Verification items for the finished model (mm, model axes). Face numbers are marked on the shaded views. A direction names the side the tool comes from. Give positions to 0.01 mm unless a question says otherwise; leave off trailing zeros. Write each loop counter-clockwise with the first axis right and the second up, starting at its lowest first coordinate (ties: lowest second). Pieces come first, ordered by that corner, then holes. Notation, with made-up numbers: M 38,-14.75 L 75,-14.75 A22 cw 75,5.25 Z; hole C 16,38.25 d6. An arc over 180 degrees is marked long. Answer as a JSON object with one key per item and string values.
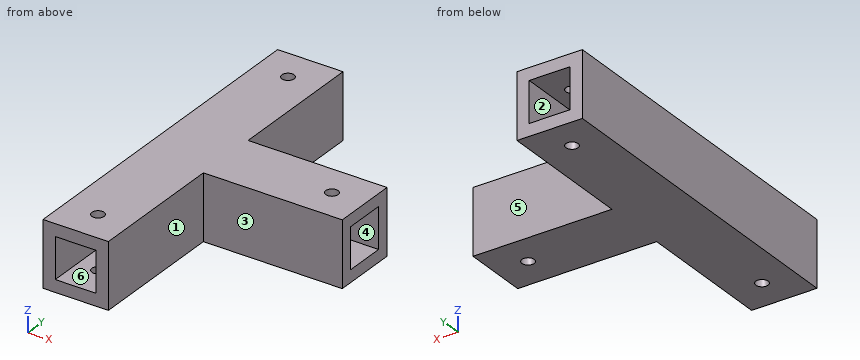
```python
from build123d import *

# Parameters (mm, degrees)
F0_W     = 16
F0_H     = 34
F1_DEPTH = 16
F2_W     = 10
F2_H     = 10
F3_DEPTH = 30
F4_W     = 10
F4_H     = 10
F5_DEPTH = 84
F6_R     = 1.5
F7_DEPTH = 16


with BuildPart() as f1:
    # F0 (on Top) → F1 (new body)
    with BuildSketch(Plane.XY):
        with Locations((-17, 33)):
            Rectangle(F0_W, F0_H)
        Polygon((-9, 16), (-25, 16), (-25, 0), (-9, 0), (25, 0), (25, 16), align=None)
        with Locations((-17, -17)):
            Rectangle(F0_W, F0_H)
    extrude(amount=F1_DEPTH)

    # F2 (on face) → F3 (cut)
    with BuildSketch(Plane.YZ.offset(25)):
        with Locations((8, 8)):
            Rectangle(F2_W, F2_H)
    extrude(amount=-F3_DEPTH, mode=Mode.SUBTRACT)

    # F4 (on face) → F5 (cut)
    with BuildSketch(Plane.XZ.offset(34)):
        with Locations((-17, 8)):
            Rectangle(F4_W, F4_H)
    extrude(amount=-F5_DEPTH, mode=Mode.SUBTRACT)

    # F6 (on face) → F7 (cut)
    with BuildSketch(Plane(origin=(0, 0, 0), x_dir=(1, 0, 0), z_dir=(0, 0, -1))):
        with Locations((-17, -42)):
            Circle(F6_R)
        with Locations((17, -8)):
            Circle(F6_R)
        with Locations((-17, 26)):
            Circle(F6_R)
    extrude(amount=-F7_DEPTH, mode=Mode.SUBTRACT)


solid = f1.part
```
1) Release check for a two-part mould opening along X. For the marked faces 1, 2 and 3 record: pulls with the +X half, pulls with the -X half, needs draft (parallel to the pull), parting line crosses it, or undercut.
Completed:
{"face 1": "pulls with the +X half", "face 2": "undercut", "face 3": "needs draft"}
2) Access from +Z, -Z, +X, -X, +Y, -Y to the whole of each face (thin tool, end or side, straight path). Record for the marked faces 4, 5 and 6.
Completed:
{"face 4": "+X", "face 5": "+Z, -Z, +X, +Y", "face 6": "+Y, -Y"}
3) Section check D-D on y = -3. Record the boundary of the cut face in (x, z), and give its area (3 significant figures).
Completed:
{"outline": "M -25,0 L -9,0 L -9,16 L -25,16 Z; hole M -22,3 L -12,3 L -12,13 L -22,13 Z", "area": "156 mm2"}
4) Section check B-B on y = 42. Record the boundary of the cut face in (x, z).
Completed:
{"outline": "M -25,0 L -18.5,0 L -18.5,3 L -22,3 L -22,13 L -18.5,13 L -18.5,16 L -25,16 Z; M -15.5,0 L -9,0 L -9,16 L -15.5,16 L -15.5,13 L -12,13 L -12,3 L -15.5,3 Z"}
5) Section check C-C on x = -17. Record the boundary of the cut face in (y, z), and give its area (3 significant figures).
Completed:
{"outline": "M -34,0 L -27.5,0 L -27.5,3 L -34,3 Z; M -34,13 L -27.5,13 L -27.5,16 L -34,16 Z; M -24.5,0 L 40.5,0 L 40.5,3 L -24.5,3 Z; M -24.5,13 L 40.5,13 L 40.5,16 L -24.5,16 Z; M 43.5,0 L 50,0 L 50,3 L 43.5,3 Z; M 43.5,13 L 50,13 L 50,16 L 43.5,16 Z", "area": "468 mm2"}
6) Go/stop test with flat-tipped pins: pin 1 (2.5 mm diameter, centred on x = -17, y = 42, fed in from -Z); pin 2 (4 mm diameter, centred on y = 40, z = 9.5, fed in from +X); pin 3 (5 mm diameter, centred on x = 12, z = 7, fed in from +Y); pin 4 (5 mm diameter, centred on y = 7, z = 7, fed in from +X). Record where each tip stops, or that it passes through.
Completed:
{"pin 1": "passes through", "pin 2": "stops at x = -9", "pin 3": "stops at y = 16", "pin 4": "stops at x = -5"}
7) Section check A-A on x = 17. Record the boundary of the cut face in (y, z).
Completed:
{"outline": "M 0,0 L 6.5,0 L 6.5,3 L 3,3 L 3,13 L 6.5,13 L 6.5,16 L 0,16 Z; M 9.5,0 L 16,0 L 16,16 L 9.5,16 L 9.5,13 L 13,13 L 13,3 L 9.5,3 Z"}
8) Thickness scan on L1, parallel to Y at x = -17, z = 1.85; L2, parallel to X at y = -27, z = 9.75; L3, parallel to Y at x = 1, z = 3.5. Record the ranges inside material, lowest first.
Completed:
{"L1": "y = -34 to -27.5, -24.5 to 40.5, 43.5 to 50", "L2": "x = -25 to -22, -12 to -9", "L3": "y = 0 to 3, 13 to 16"}
